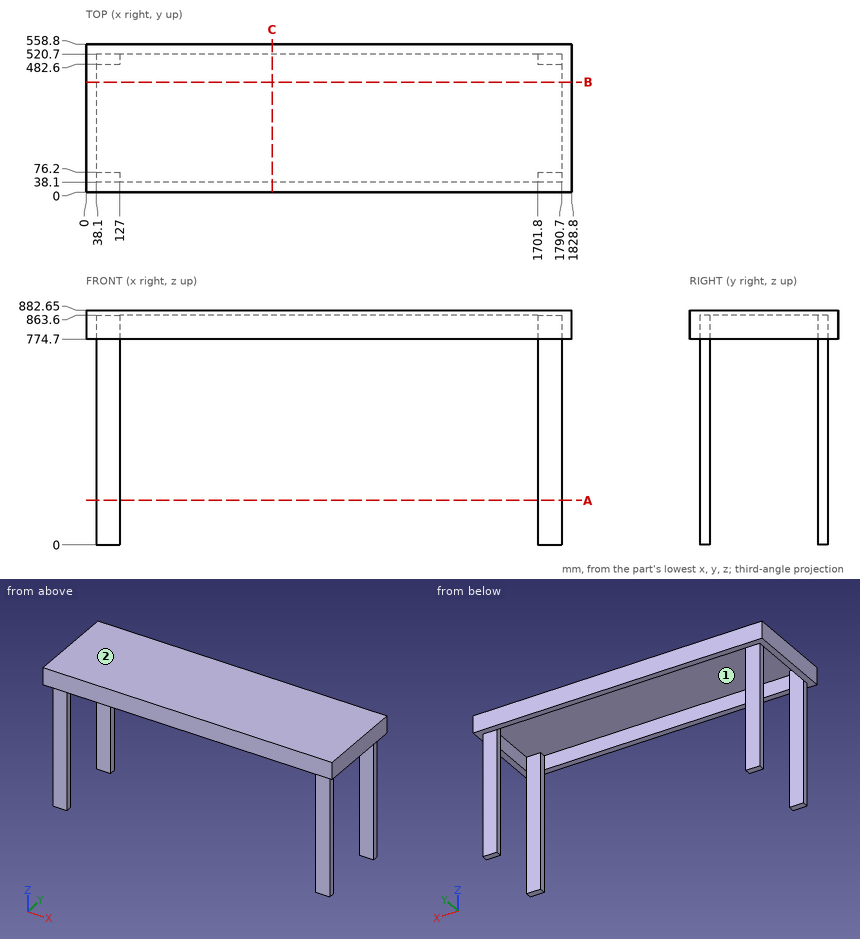
Check sheet for the drawn part. Datum: minimum x, y, z corner. Units: mm. Round coordinates to 2 decimals unless told otherwise and drop trailing zeros. Order: outer loops, then holes, each group sorted by start corner. A loop starts at its lowest first (then second) coordinate and runs counter-clockwise, first axis right, second up.
(1) Draft check along X on the marked faces 1 and 2. Enter one of: pulls with the +X half, pulls with the -X half, needs draft (parallel to the pull), parting line crosses it, or undercut.
(2) Cross-section at C-C, the plane x = 701. Enter the section's corners in (y, z).
(3) Go/stop test with flat-tipped pins: P1, Ø4, axis at x = 481, y = 466, coming from the -Z side; P2, Ø6, axis at y = 185, z = 792.5, coming from the -X side; P3, Ø12, axis at y = 498, z = 687.5, coming from the +X side; P4, Ø19, axis at y = 51, z = 539.5, coming from the -X side. Record where each tip stops, or that it passes through.
(4) Cross-section at B-B, the plane y = 415. Enter the section's corners in (x, z).
(5) Cross-section at A-A, the plane z = 167. Enter the section's corners in (x, y), and give its area (3 significant figures).
(6) Scan lines: probe 1 along X at (y, z) = (415, 784); probe 2 along Y at (x, z) = (97, 177); probe 3 along Z at (x, y) = (1595.5, 296). Record each from-to range of solid material in increasing order.
Check sheet entries:
1. face 1: undercut
1. face 2: needs draft
2. outline: (0, 774.7) - (38.1, 774.7) - (38.1, 863.6) - (520.7, 863.6) - (520.7, 774.7) - (558.8, 774.7) - (558.8, 882.65) - (0, 882.65) - close
3. P1: stops at z = 863.6
3. P2: stops at x = 0
3. P3: stops at x = 1790.7
3. P4: stops at x = 38.1
4. outline: (0, 774.7) - (38.1, 774.7) - (38.1, 863.6) - (1790.7, 863.6) - (1790.7, 774.7) - (1828.8, 774.7) - (1828.8, 882.65) - (0, 882.65) - close
5. outline: (38.1, 38.1) - (127, 38.1) - (127, 76.2) - (38.1, 76.2) - close; (38.1, 482.6) - (127, 482.6) - (127, 520.7) - (38.1, 520.7) - close; (1701.8, 38.1) - (1790.7, 38.1) - (1790.7, 76.2) - (1701.8, 76.2) - close; (1701.8, 482.6) - (1790.7, 482.6) - (1790.7, 520.7) - (1701.8, 520.7) - close
5. area: 13,500 mm2
6. probe 1: x = 0 to 38.1, 1790.7 to 1828.8
6. probe 2: y = 38.1 to 76.2, 482.6 to 520.7
6. probe 3: z = 863.6 to 882.65
